Verification items for this drawing (mm, ordinates from the low corner). A direction names the side the tool comes from. Round coordinates to 2 decimals unless told otherwise and drop trailing zeros. Loops run counter-clockwise (first coordinate to the right, second up) from the corner with the lowest first, then second, coordinate; pieces in that order, holes last. Notation, with made-up numbers: M 22.25,39 L 42.25,39 A22 ccw 42.25,77 Z; hole C 23.5,29.5 d7. An arc over 180 degrees is marked long. One line per item, written item: value.
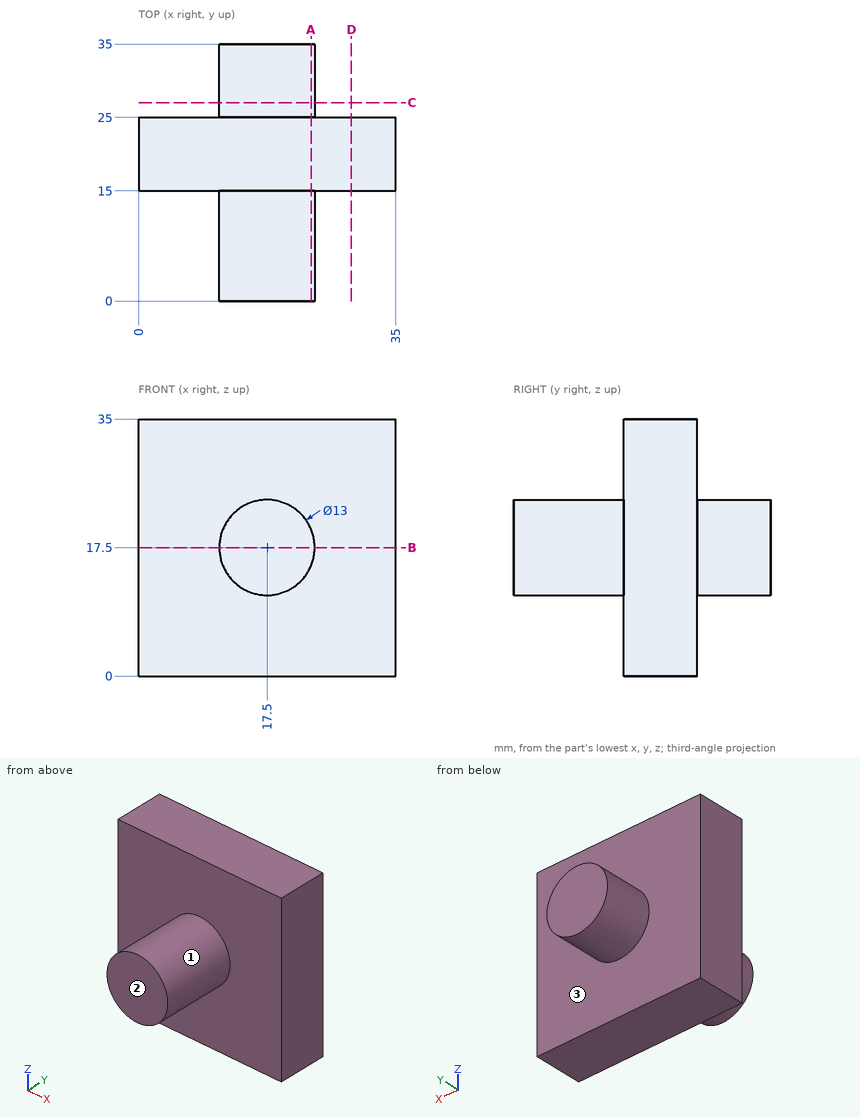
(1) Thickness scan on L1, parallel to Y at x = 22, z = 24.5; L2, parallel to Z at x = 18, y = 2; L3, parallel to Z at x = 22, y = 28. Record the ranges inside material, lowest first. Write a range as from..to.
Completed:
L1: y = 15..25
L2: z = 11.02..23.98
L3: z = 12.81..22.19
(2) Sectioned sample at A-A on x = 23.5. Enter the section's corners in (y, z).
Completed:
outline: M 0,15 L 15,15 L 15,0 L 25,0 L 25,15 L 35,15 L 35,20 L 25,20 L 25,35 L 15,35 L 15,20 L 0,20 Z
(3) Sectioned sample at D-D on x = 29. Enter the section's corners in (y, z), and give its area (3 significant figures).
Completed:
outline: M 15,0 L 25,0 L 25,35 L 15,35 Z
area: 350 mm^2
(4) Sectioned sample at C-C on y = 27. Enter the section's corners in (x, z).
Completed:
outline: C 17.5,17.5 d13
(5) Tool access check on the marked faces 1, 2 and 3. Record the directions out of +Z, -Z, +X, -X, +Y, -Y that give a thin tool (end or side, any length) a straight path to the whole face; none if there is none.
Completed:
face 1: -Y
face 2: +Z, -Z, +X, -X, -Y
face 3: +Y
(6) Sectioned sample at B-B on z = 17.5. Enter the section's corners in (x, y).
Completed:
outline: M 0,15 L 11,15 L 11,0 L 24,0 L 24,15 L 35,15 L 35,25 L 24,25 L 24,35 L 11,35 L 11,25 L 0,25 Z
(7) Depth check by flat-ended pin: pin 1 Ø5 at (x, y) = (12.5, 8.5) entering from +Z; pin 2 Ø4 at (x, z) = (24, 5.5) entering from +Y; pin 3 Ø10 at (x, y) = (26, 5) entering from +Z. Enter the tip coordinate at first touch or a pass-through.
Completed:
pin 1: stops at z = 23.5
pin 2: stops at y = 25
pin 3: stops at z = 22.98
